Read the model definition and answer for the solid it produces. Units are mm, in the model's axes. Coordinates: 2 decimals unless noted, no trailing zeros. Order: outer loops, then holes, each group sorted by start corner. A loop starts at its lowest first (then second) coordinate and runs counter-clockwise, first axis right, second up. Notation, with made-up numbers: M 36,-30 L 45,-30 A11 cw 45,-26 Z; hole C -10,-2 d4. An arc over 180 degrees is marked long. Put each result on its own line as item: value.
Autodesk Inventor part; units mm, degrees
ref_plane "YZ Plane" through (0, 0, 0) normal (1, 0, 0) x (0, 1, 0)
ref_plane "XZ Plane" through (0, 0, 0) normal (0, 1, 0) x (-1, 0, 0)
ref_plane "XY Plane" through (0, 0, 0) normal (0, 0, 1) x (1, 0, 0)
sketch "Sketch1" plane through (0, 0, 0) normal (0, 1, 0) x (-1, 0, 0)
  arc A0 (0, -177) -> (0, 177) centre (0, 0) ccw
  line L0 (0, 177) -> (-151.6, 177)
  line L1 (-177, 151.6) -> (-177, -151.6)
  line L2 (-151.6, -177) -> (0, -177)
  arc A1 (-151.6, 177) -> (-177, 151.6) centre (-151.6, 151.6) ccw
  arc A2 (-177, -151.6) -> (-151.6, -177) centre (-151.6, -151.6) ccw
  point P0 (-177, 177)
  point P1 (-177, -177)
  dimension "d0" = 354
  dimension "d1" = 177
  dimension "d2" = 177
  dimension "d115" = 25.4
  dimension "d116" = 25.4
extrude "Extrusion1" add sketch "Sketch1" along normal blind 5
sketch "Sketch2" plane through (0, 5, 0) normal (0, 1, 0) x (1, 0, 0)
  circle A0 centre (-51.435, -34.125) radius 1.7
  circle A1 centre (-51.435, 34.125) radius 1.7
  circle A2 centre (51.435, 34.125) radius 1.7
  circle A3 centre (51.435, -34.125) radius 1.7
  line L0 (0, -177) -> (151.6, -177) construction
  line L1 (151.6, 177) -> (0, 177) construction
  line L2 (0, -177) -> (0, 177) construction
  arc A4 (0, 177) -> (0, -177) centre (0, 0) ccw construction
  line L3 (-177, 0) -> (177, 0) construction
  line L4 (177, -151.6) -> (177, 151.6) construction
  circle A5 centre (26.035, 59.5249) radius 1.7
  circle A6 centre (26.035, -59.5249) radius 1.7
  circle A7 centre (-26.035, 59.5249) radius 1.7
  circle A8 centre (-26.035, -59.5249) radius 1.7
  point P0 (177, -177)
  point P1 (177, 177)
  dimension "d5" = 3.4
  dimension "d6" = 3.4
  dimension "d8" = 3.4
  dimension "d10" = 3.4
  dimension "d12" = 68.25
  dimension "d13" = 68.25
  dimension "d14" = 102.87
  dimension "d15" = 102.87
  dimension "d18" = 51.435
  dimension "d19" = 51.435
  dimension "d20" = 34.125
  dimension "d21" = 34.125
  dimension "d153" = 3.4
  dimension "d155" = 3.4
  dimension "d157" = 3.4
  dimension "d159" = 3.4
  dimension "d161" = 52.07
  dimension "d162" = 26.035
  dimension "d163" = 52.07
  dimension "d164" = 26.035
  dimension "d165" = 119.0498
  dimension "d166" = 119.0498
  dimension "d167" = 59.5249
  dimension "d168" = 59.5249
extrude "Jetson Holes" cut sketch "Sketch2" against normal through all
sketch "Sketch3" plane through (0, 5, 0) normal (0, 1, 0) x (1, 0, 0)
  circle A0 centre (-12.7, -63.5) radius 9.525
  arc A1 (0, 177) -> (0, -177) centre (0, 0) ccw construction
  line L0 (177, -151.6) -> (177, 151.6) construction
  line L1 (151.6, 177) -> (0, 177) construction
  line L2 (0, -177) -> (151.6, -177) construction
  line L3 (0, 177) -> (0, -177) construction
  line L4 (177, 0) -> (-177, 0) construction
  point P0 (177, -177)
  point P1 (177, 177)
  dimension "d24" = 19.05
  dimension "d26" = 63.5
  dimension "d27" = 12.7
extrude "SPI_Holes" cut sketch "Sketch3" against normal through all
sketch "Sketch4" plane through (0, 5, 0) normal (0, 1, 0) x (1, 0, 0)
  circle A0 centre (-60.96, -76.2) radius 1.7
  circle A1 centre (60.96, -101.6) radius 1.7
  circle A2 centre (60.96, 76.2) radius 1.7
  circle A3 centre (-60.96, 101.6) radius 1.7
  line L0 (177, -151.6) -> (177, 151.6) construction
  line L1 (177, 0) -> (-177, 0) construction
  arc A4 (0, 177) -> (0, -177) centre (0, 0) ccw construction
  line L2 (151.6, 177) -> (0, 177) construction
  line L3 (0, -177) -> (151.6, -177) construction
  line L4 (0, -177) -> (0, 177) construction
  circle A5 centre (-12.7, -63.5) radius 9.525 construction
  circle A6 centre (-101.6, 50.8) radius 8.89
  circle A7 centre (-101.6, -50.8) radius 8.89
  circle A8 centre (41.91, -76.2) radius 1.7
  circle A9 centre (-41.91, -101.6) radius 1.7
  circle A10 centre (-41.91, 76.2) radius 1.7
  circle A11 centre (41.91, 101.6) radius 1.7
  point P0 (177, -177)
  point P1 (177, 177)
  dimension "d30" = 3.4
  dimension "d31" = 3.4
  dimension "d33" = 3.4
  dimension "d35" = 3.4
  dimension "d37" = 121.92
  dimension "d38" = 121.92
  dimension "d39" = 25.4
  dimension "d40" = 25.4
  dimension "d41" = 60.96
  dimension "d42" = 60.96
  dimension "d43" = 12.7
  dimension "d44" = 177.8
  dimension "d45" = 17.78
  dimension "d46" = 17.78
  dimension "d47" = 50.8
  dimension "d48" = 50.8
  dimension "d49" = 101.6
  dimension "d50" = 101.6
  dimension "d139" = 3.4
  dimension "d140" = 19.05
  dimension "d141" = 25.4
  dimension "d142" = 3.4
  dimension "d143" = 19.05
  dimension "d144" = 25.4
  dimension "d145" = 3.4
  dimension "d147" = 3.4
  dimension "d149" = 25.4
  dimension "d150" = 25.4
  dimension "d151" = 19.05
  dimension "d152" = 19.05
extrude "NiMH Holes" cut sketch "Sketch4" against normal through all
sketch "Sketch5" plane through (0, 5, 0) normal (0, 1, 0) x (1, 0, 0)
  circle A0 centre (-8.1625, 9.55) radius 1.7
  circle A1 centre (-8.1625, -9.55) radius 1.7
  circle A2 centre (8.1625, -9.55) radius 1.7
  circle A3 centre (8.1625, 9.55) radius 1.7
  arc A4 (0, 177) -> (0, -177) centre (0, 0) ccw construction
  line L0 (0, -177) -> (0, 177) construction
  line L1 (-177, 0) -> (177, 0)
  line L2 (177, -151.6) -> (177, 151.6)
  point P0 (177, -177)
  point P1 (177, 177)
  dimension "d53" = 3.4
  dimension "d54" = 3.4
  dimension "d56" = 3.4
  dimension "d58" = 3.4
  dimension "d60" = 16.325
  dimension "d61" = 16.325
  dimension "d62" = 19.1
  dimension "d63" = 19.1
  dimension "d64" = 8.1625
  dimension "d65" = 8.1625
  dimension "d66" = 9.55
  dimension "d67" = 9.55
extrude "IMU Holes" cut sketch "Sketch5" against normal through all
sketch "Sketch8" plane through (0, 5, 0) normal (0, 1, 0) x (1, 0, 0)
  circle A0 centre (-101.6, 101.6) radius 1.7
  circle A1 centre (-101.6, -101.6) radius 1.7
  circle A2 centre (101.6, -101.6) radius 1.7
  circle A3 centre (101.6, 101.6) radius 1.7
  line L0 (177, -151.6) -> (177, 151.6) construction
  line L1 (177, 0) -> (-177, 0) construction
  arc A4 (0, 177) -> (0, -177) centre (0, 0) ccw construction
  line L2 (151.6, 177) -> (0, 177) construction
  line L3 (0, -177) -> (151.6, -177) construction
  line L4 (0, 177) -> (0, -177) construction
  circle A5 centre (101.6, 0) radius 1.7
  point P0 (177, -177)
  point P1 (177, 177)
  dimension "d97" = 3.4
  dimension "d98" = 3.4
  dimension "d100" = 3.4
  dimension "d102" = 3.4
  dimension "d104" = 101.6
  dimension "d105" = 101.6
  dimension "d106" = 101.6
  dimension "d107" = 101.6
  dimension "d108" = 101.6
  dimension "d109" = 101.6
  dimension "d110" = 101.6
  dimension "d111" = 101.6
  dimension "d169" = 3.4
  dimension "d170" = 101.6
extrude "Level1 Standoffs" cut sketch "Sketch8" against normal through all
sketch "Sketch6" plane through (0, 5, 0) normal (0, 1, 0) x (1, 0, 0)
  circle A0 centre (-82.55, -114.3) radius 1.7
  circle A1 centre (-82.55, 114.3) radius 1.7
  circle A2 centre (82.55, 114.3) radius 1.7
  circle A3 centre (82.55, -114.3) radius 1.7
  arc A4 (0, 177) -> (0, -177) centre (0, 0) ccw construction
  line L0 (177, -151.6) -> (177, 151.6) construction
  line L1 (0, -177) -> (151.6, -177) construction
  line L2 (0, 178.2067) -> (0, -177) construction
  line L3 (-177, 0) -> (177, 0) construction
  point P0 (177, -177)
  point P1 (177, 177)
  dimension "d70" = 3.4
  dimension "d71" = 3.4
  dimension "d73" = 3.4
  dimension "d75" = 3.4
  dimension "d77" = 82.55
  dimension "d80" = 82.55
  dimension "d81" = 82.55
  dimension "d84" = 82.55
  dimension "d85" = 114.3
  dimension "d86" = 114.3
  dimension "d87" = 114.3
  dimension "d88" = 114.3
extrude "Level3 Standoffs" cut sketch "Sketch6" against normal through all
sketch "Sketch7" plane through (0, 5, 0) normal (0, 1, 0) x (1, 0, 0)
  line L0 (177, -151.6) -> (177, 151.6) construction
  line L1 (177, 0) -> (-177, 0) construction
  arc A0 (0, 177) -> (0, -177) centre (0, 0) ccw construction
  circle A1 centre (-141.44, 0) radius 2.667
  line L2 (0, 177) -> (0, -177) construction
  circle A2 centre (-114.4274, -83.1363) radius 2.667
  circle A3 centre (-114.4274, 83.1363) radius 2.667
  circle A4 centre (-43.7074, -134.5174) radius 2.667
  circle A5 centre (-43.7074, 134.5174) radius 2.667
  circle A6 centre (38.1, -141.44) radius 2.667
  line L3 (0, -177) -> (151.6, -177)
  circle A7 centre (114.3, -141.44) radius 2.667
  circle A8 centre (38.1, 141.44) radius 2.667
  circle A9 centre (114.3, 141.44) radius 2.667
  circle A10 centre (141.44, 101.6) radius 2.667
  circle A11 centre (141.44, 0) radius 2.667
  circle A12 centre (141.44, -101.6) radius 2.667
  arc A13 (151.6, -177) -> (177, -151.6) centre (151.6, -151.6) ccw construction
  line L4 (177, -151.6) -> (177, 151.6) construction
  line L5 (151.6, 177) -> (0, 177) construction
  point P0 (177, -177)
  point P1 (177, 177)
  point P2 (-177, 0)
  dimension "d91" = 5.334
  dimension "d92" = 35.56
  dimension "d95" = 144
  dimension "d114" = 5.334
  dimension "d117" = 35.56
  dimension "d118" = 5.334
  dimension "d119" = 5.334
  dimension "d120" = 5.334
  dimension "d121" = 5.334
  dimension "d122" = 5.334
  dimension "d123" = 5.334
  dimension "d124" = 35.56
  dimension "d125" = 35.56
  dimension "d126" = 35.56
  dimension "d127" = 35.56
  dimension "d128" = 35.56
  dimension "d129" = 35.56
  dimension "d130" = 38.1
  dimension "d132" = 38.1
  dimension "d133" = 101.6
  dimension "d134" = 101.6
  dimension "d135" = 76.2
  dimension "d136" = 76.2
extrude "Zip Ties" cut sketch "Sketch7" against normal through all
sketch "Sketch9" plane through (0, 5, 0) normal (0, 1, 0) x (1, 0, 0)
  circle A0 centre (-110.89, 17.1) radius 1.7
  circle A1 centre (-110.89, -17.1) radius 1.7
  circle A2 centre (-135.09, 17.1) radius 1.7
  line L0 (0, 0) -> (-177, 0) construction
  arc A3 (0, 177) -> (0, -177) centre (0, 0) ccw construction
  circle A4 centre (-141.44, 0) radius 2.667 construction
  dimension "d171" = 3.4
  dimension "d172" = 3.4
  dimension "d174" = 3.4
  dimension "d176" = 24.2
  dimension "d177" = 34.2
  dimension "d178" = 17.1
  dimension "d179" = 6.35
  dimension "d180" = 17.1
  dimension "d181" = 17.1
extrude "Mic_MCU_Case" cut sketch "Sketch9" against normal blind 25.4
sketch "Sketch10" plane through (0, 5, 0) normal (0, 1, 0) x (1, 0, 0)
  circle A0 centre (88.9, 0) radius 1.7
  point P0 (0, 0)
  dimension "d184" = 3.4
  dimension "d185" = 88.9
extrude "Extrusion10" cut sketch "Sketch10" against normal blind 25.4
equation "\"d0\" = robot_diameter"
equation "\"d3\" = hardboard_thickness"
equation "\"d5\" = m3_clearance"
equation "\"d6\" = d7"
equation "\"d8\" = d9"
equation "\"d10\" = d11"
equation "\"d13\" = d12"
equation "\"d19\" = d18"
equation "\"d20\" = d21"
equation "\"d21\" = 0.5 * d12"
equation "\"d153\" = d154"
equation "\"d155\" = d156"
equation "\"d157\" = d158"
equation "\"d159\" = d160"
equation "\"d162\" = 0.5 * d161"
equation "\"d163\" = d161"
equation "\"d164\" = d162"
equation "\"d166\" = d165"
equation "\"d167\" = 0.5 * d165"
equation "\"d168\" = d167"
equation "\"d30\" = m3_clearance"
equation "\"d31\" = d32"
equation "\"d33\" = d34"
equation "\"d35\" = d36"
equation "\"d38\" = d37"
equation "\"d40\" = d39"
equation "\"d41\" = 0.5 * d37"
equation "\"d42\" = 0.5 * d38"
equation "\"d46\" = d45"
equation "\"d48\" = d47"
equation "\"d50\" = d49"
equation "\"d139\" = m3_clearance"
equation "\"d141\" = d40"
equation "\"d142\" = m3_clearance"
equation "\"d144\" = d40"
equation "\"d145\" = d146"
equation "\"d147\" = d148"
equation "\"d149\" = d39"
equation "\"d150\" = d39"
equation "\"d152\" = d151"
equation "\"d53\" = m3_clearance"
equation "\"d54\" = d55"
equation "\"d56\" = d57"
equation "\"d58\" = d59"
equation "\"d61\" = d60"
equation "\"d63\" = d62"
equation "\"d64\" = 0.5 * d60"
equation "\"d65\" = d64"
equation "\"d66\" = 0.5 * d63"
equation "\"d67\" = d66"
equation "\"d97\" = m3_clearance"
equation "\"d98\" = d99"
equation "\"d100\" = d101"
equation "\"d102\" = d103"
equation "\"d106\" = d105"
equation "\"d107\" = d104"
equation "\"d108\" = d104"
equation "\"d109\" = d104"
equation "\"d110\" = d105"
equation "\"d111\" = d105"
equation "\"d169\" = m3_clearance"
equation "\"d70\" = m3_clearance"
equation "\"d71\" = d72"
equation "\"d73\" = d74"
equation "\"d75\" = d76"
equation "\"d80\" = d77"
equation "\"d81\" = d77"
equation "\"d84\" = d77"
equation "\"d86\" = d85"
equation "\"d87\" = d85"
equation "\"d88\" = d85"
equation "\"d117\" = d124"
equation "\"d124\" = d92"
equation "\"d125\" = d124"
equation "\"d126\" = d124"
equation "\"d127\" = d124"
equation "\"d128\" = d124"
equation "\"d129\" = d124"
equation "\"d132\" = d130"
equation "\"d171\" = m3_clearance"
equation "\"d172\" = d173"
equation "\"d174\" = d175"
equation "\"d178\" = 0.5 * d177"
equation "\"d180\" = d178"
equation "\"d181\" = d178"
equation "\"d184\" = m3_clearance"
equation "\"m3_heat_set_insert\" = 4"
equation "\"m3_clearance\" = 3.4"
equation "\"m3_heat_set_depth\" = 7"
equation "\"robot_diameter\" = 354"
equation "\"hardboard_thickness\" = 5"
equation "\"motor_centerline_height\" = 13"
properties part number "layer2_new"
Q1. Consider line 1 along Z through (x, y) = (41.91, 2.3); line 2 along Z through (x, y) = (84, 2.6); line 3 along X through (y, z) = (0.2, 143). Determine where each line is inside the solid, lowest interval first.
Answers below:
line 1: z = -177 to -103.3, -99.9 to 74.5, 77.9 to 177
line 2: z = -177 to -115.19, -113.41 to 113.41, 115.19 to 177
line 3: x = -104.31 to 35.94, 40.26 to 112.14, 116.46 to 177
Q2. For a pull along X with two mould halves and no side action, classify faces 1 (the face through (-110.48, 2.54, -51.19)), 2 (the face through (2, 0, 2)), 3 (the face through (169.76, 2.46, 169.36)) as +X half, -X half, draft (parallel to the pull), parting line (faces both ways), or undercut.
Answers below:
face 1: undercut
face 2: draft
face 3: +X half
Q3. Find section A-A on y = 1.2. Give the number of separate pieces and of enclosed holes in the cut face, plus the area to 3 significant figures.
Answers below:
separate pieces: 1
enclosed holes: 48
area: 110,000 mm^2
Q4. Given pin 1 (4 mm diameter, centred on x = -101.6, z = -101.6, fed in from +Y); pin 2 (5 mm diameter, centred on x = 114.3, z = 141.44, fed in from +Y); pin 3 (1.5 mm diameter, centred on x = -85, y = 1, fed in from +Z); pin 4 (1 mm diameter, centred on x = -14, y = 2, fed in from -Z), each flat-ended and moving along its own axis, determine where each tip first touches the part or whether it passes through.
Answers below:
pin 1: stops at y = 5
pin 2: passes through
pin 3: stops at z = 155.66
pin 4: stops at z = -176.48
Q5. Find section B-B on z = 126. Write down the section's boundary in (x, y), plus the area to 3 significant figures.
Answers below:
outline: M -124.31,0 L 177,0 L 177,5 L -124.31,5 Z
area: 1,510 mm^2
